Geometry check sheet. Reference: the model listing, model coordinates, mm. Face numbers are marked on the shaded views. A direction names the side the tool comes from. Round coordinates to 2 decimals unless told otherwise and drop trailing zeros. Order: outer loops, then holes, each group sorted by start corner. A loop starts at its lowest first (then second) coordinate and runs counter-clockwise, first axis right, second up. Notation, with made-up numbers: (27.25, 31) - (85.25, 31) arc R27 cw to (85.25, 62) - close; hole circle Ø4 at (-3, 70.25). An arc over 180 degrees is marked (long way). One line per question, with ' | ' between items. Start each with the question number.
Q1. Sectioned sample at C-C, the plane x = -3. Enter the section's corners in (y, z).
Q2. Sectioned sample at A-A, the plane x = 0. Enter the section's corners in (y, z), then the cut area to 3 significant figures.
Q3. Sectioned sample at D-D, the plane y = -3.25. Enter the section's corners in (x, z), then the cut area to 3 significant figures.
Q4. Tool access check on the marked faces 5, 6, 7 and 8. Record the directions out of +Z, -Z, +X, -X, +Y, -Y that give a thin tool (end or side, any length) a straight path to the whole face; none if there is none.
Q5. Mould release check, pull along Z, two halves, no side actions. Record for the marked faces 1, 2, 3 and 4: +Z half, -Z half, draft (parallel to the pull), parting line (faces both ways), or undercut.
Q6. Gauge pin test, flat ends, axial feed: P1, Ø1.5, axis at y = -2.5, z = 13, coming from the -X side; P2, Ø2, axis at y = 2, z = 26, coming from the +X side; P3, Ø1.5, axis at x = -0.5, z = 8.5, coming from the +Y side. Record the tip position at first contact, or that the pin passes through.
Q7. Material ranges on line 1 along Z through (x, y) = (-1, -3.25); line 2 along X through (y, z) = (0.75, 12); line 3 along X through (y, z) = (-1.75, 24), recorded low to high.
Autodesk Inventor part; units mm, degrees
ref_plane "YZ Plane" through (0, 0, 0) normal (1, 0, 0) x (0, 1, 0)
ref_plane "XZ Plane" through (0, 0, 0) normal (0, 1, 0) x (-1, 0, 0)
ref_plane "XY Plane" through (0, 0, 0) normal (0, 0, 1) x (1, 0, 0)
sketch "Эскиз1" plane through (0, 0, 0) normal (0, 0, 1) x (1, 0, 0)
  circle A0 centre (0, 0) radius 2
  dimension "d0" = 4
extrude "Выдавливание1" add sketch "Эскиз1" along normal blind 10
sketch "Эскиз2" plane through (0, 0, 10) normal (0, 0, 1) x (1, 0, 0)
  circle A0 centre (0, 0) radius 4
  dimension "d5" = 8
extrude "Выдавливание2" add sketch "Эскиз2" along normal blind 0.5
mirror "Зеркальное отражение1" about plane through (0, 0, 10.5) normal (0, 0, 1) of "Выдавливание2", "Выдавливание1"
sketch "Эскиз3" plane through (0, 0, 21) normal (0, 0, 1) x (1, 0, 0)
  circle A0 centre (-7.3376, 4.7247) radius 20.8096
  point P0 (0, 0)
extrude "Выдавливание3" cut sketch "Эскиз3" against normal blind 5
mirror "Зеркальное отражение3" about plane through (-7.3376, 4.7247, 16) normal (0, 0, 1)
thread "Резьба4"
properties part number "ось крепление пушки" material "Железо, ковкое"
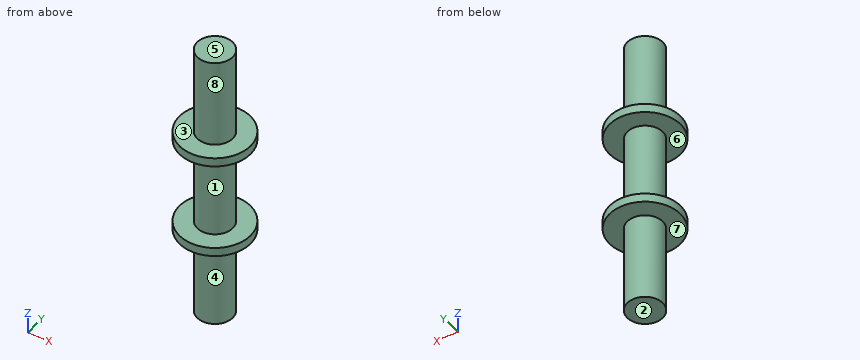
Determined:
1) outline: (-2.65, 10) - (2.65, 10) - (2.65, 11) - (-2.65, 11) - close; (-2.65, 21) - (2.65, 21) - (2.65, 22) - (-2.65, 22) - close
2) outline: (-4, 10) - (-2, 10) - (-2, 0) - (2, 0) - (2, 10) - (4, 10) - (4, 11) - (2, 11) - (2, 21) - (4, 21) - (4, 22) - (2, 22) - (2, 32) - (-2, 32) - (-2, 22) - (-4, 22) - (-4, 21) - (-2, 21) - (-2, 11) - (-4, 11) - close | area: 136 mm2
3) outline: (-2.33, 10) - (2.33, 10) - (2.33, 11) - (-2.33, 11) - close; (-2.33, 21) - (2.33, 21) - (2.33, 22) - (-2.33, 22) - close | area: 9.33 mm2
4) face 5: +Z, +X, -X, +Y, -Y | face 6: none | face 7: -Z | face 8: +Z
5) face 1: undercut | face 2: -Z half | face 3: +Z half | face 4: draft
6) P1: stops at x = -0.97 | P2: stops at x = 1.73 | P3: stops at y = 2
7) line 1: z = 10 to 11, 21 to 22 | line 2: x = -1.85 to 1.85 | line 3: x = -0.97 to 0.97
